Can you work these out from the drawing? Everything is in mm from the part's minimum corner. Give positions to 0.01 mm unless a question says otherwise; leave off trailing zeros. Write each loop counter-clockwise with the first axis right and the second up, starting at its lowest first coordinate (ties: lowest second). Pieces come first, ordered by that corner, then holes. Notation, with made-up numbers: (35.25, -20.75) - (78.25, -20.75) arc R18 cw to (78.25, 14.25) - close; hole circle Ø6 at (76.5, -20.75). An arc over 180 degrees is marked (long way). Use a Markdown table: item, result. Add a question column.
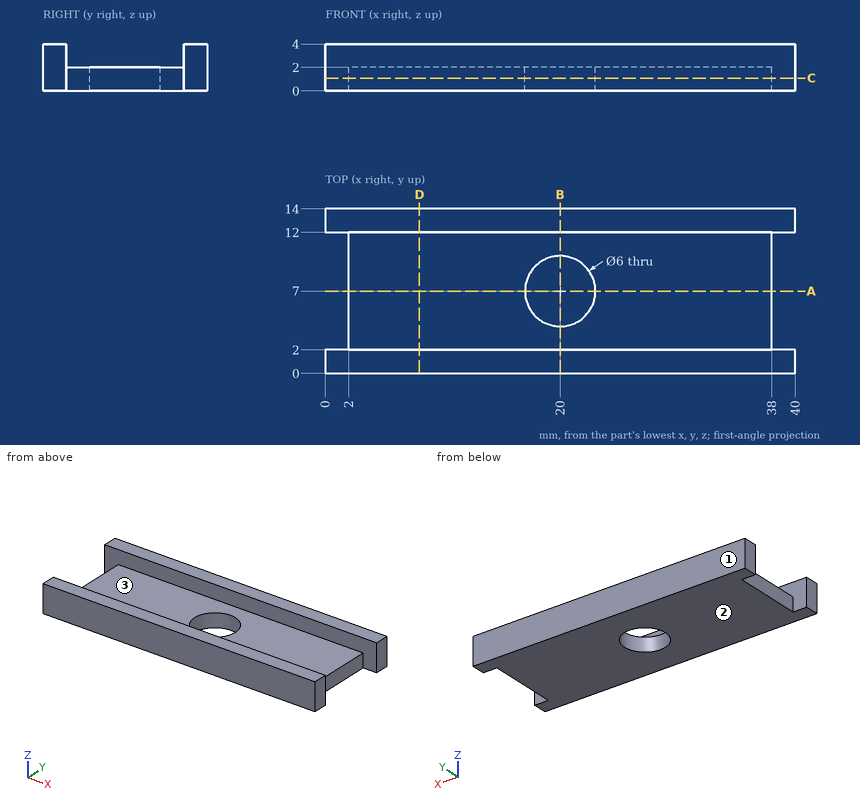
Q1. Suppose I cut it at D-D (x = 8). Please give me the cut outline in (y, z), and give its area (3 significant figures).
Q2. If we mould it in two halves opening along Y, with no side actions, what happens to the marked faces 1, 2 and 3? For each: released by +Y, released by -Y, zero draft, split by the parting line, or undercut.
Q3. Suppose I cut it at B-B (x = 20). Please give me the cut outline in (y, z), and give its area (3 significant figures).
Q4. If I drill on probe 1 along Y at (x, z) = (19, 3); probe 2 along Y at (x, z) = (20, 0.95); probe 3 along X at (y, z) = (3.25, 1.15), over which ranges is the centre line in solid material (lowest first)? Write a range as [from, to].
Q5. I'm going to push flat-ended pins straight in: P1, Ø5, axis at x = 24.5, y = 6, coming from the +Z side; P2, Ø1.6, axis at y = 4.5, z = 1.5, coming from the +X side; P3, Ø2, axis at y = 6.5, z = 0.5, coming from the -X side. Where does each tip first touch, or does it pass through?
Q6. Suppose I cut it at A-A (y = 7). Please give me the cut outline in (x, z).
Q7. Suppose I cut it at C-C (z = 1.1). Please give me the cut outline in (x, y).
Derived:
| question | item | result |
|---|---|---|
| 1 | outline | (0, 0) - (14, 0) - (14, 4) - (12, 4) - (12, 2) - (2, 2) - (2, 4) - (0, 4) - close |
| 1 | area | 36.0 mm² |
| 2 | face 1 | released by +Y |
| 2 | face 2 | zero draft |
| 2 | face 3 | undercut |
| 3 | outline | (0, 0) - (4, 0) - (4, 2) - (2, 2) - (2, 4) - (0, 4) - close; (10, 0) - (14, 0) - (14, 4) - (12, 4) - (12, 2) - (10, 2) - close |
| 3 | area | 24.0 mm² |
| 4 | probe 1 | [0, 2], [12, 14] |
| 4 | probe 2 | [0, 4], [10, 14] |
| 4 | probe 3 | [2, 38] |
| 5 | P1 | z = 2 |
| 5 | P2 | x = 38 |
| 5 | P3 | x = 2 |
| 6 | outline | (2, 0) - (17, 0) - (17, 2) - (2, 2) - close; (23, 0) - (38, 0) - (38, 2) - (23, 2) - close |
| 7 | outline | (0, 0) - (40, 0) - (40, 2) - (38, 2) - (38, 12) - (40, 12) - (40, 14) - (0, 14) - (0, 12) - (2, 12) - (2, 2) - (0, 2) - close; hole circle Ø6 at (20, 7) |
